from build123d import *

# Parameters (mm, degrees)
F0_R     = 2.75
F1_DEPTH = 7.5
F2_R     = 2


with BuildPart() as f1:
    # F0 (on Top) → F1 (new body)
    with BuildSketch(Plane.XY):
        with BuildLine():
            Line((23.5, 40), (-23.5, 40))
            ThreePointArc((-23.5, 40), (-27.035534, 38.535534), (-28.5, 35))
            Line((-28.5, 35), (-28.5, -35))
            ThreePointArc((-28.5, -35), (-27.035534, -38.535534), (-23.5, -40))
            Line((-23.5, -40), (23.5, -40))
            ThreePointArc((23.5, -40), (27.035534, -38.535534), (28.5, -35))
            Line((28.5, -35), (28.5, 35))
            ThreePointArc((28.5, 35), (27.035534, 38.535534), (23.5, 40))
        make_face()
        with Locations((-23.5, -30)):
            Circle(F0_R, mode=Mode.SUBTRACT)
        with Locations((23.5, -30)):
            Circle(F0_R, mode=Mode.SUBTRACT)
        with Locations((-23.5, 0)):
            Circle(F0_R, mode=Mode.SUBTRACT)
        with Locations((-23.5, 30)):
            Circle(F0_R, mode=Mode.SUBTRACT)
        with BuildLine():
            ThreePointArc((-18.5, 33), (-17.914214, 34.414214), (-16.5, 35))
            Line((-16.5, 35), (16.5, 35))
            ThreePointArc((16.5, 35), (17.914214, 34.414214), (18.5, 33))
            Line((18.5, 33), (18.5, -33))
            ThreePointArc((18.5, -33), (17.914214, -34.414214), (16.5, -35))
            Line((16.5, -35), (-16.5, -35))
            ThreePointArc((-16.5, -35), (-17.914214, -34.414214), (-18.5, -33))
            Line((-18.5, -33), (-18.5, 33))
        make_face(mode=Mode.SUBTRACT)
        with Locations((23.5, 0)):
            Circle(F0_R, mode=Mode.SUBTRACT)
        with Locations((23.5, 30)):
            Circle(F0_R, mode=Mode.SUBTRACT)
    extrude(amount=F1_DEPTH)

    # F2
    f2_edges = [f1.edges().sort_by_distance(p)[0] for p in [
        (-18.5, 0, 7.5),
        (0, -40, 7.5),
    ]]
    fillet(f2_edges, radius=F2_R)


solid = f1.part
Here's how the part is built. I have some questions about the finished solid (model axes, mm). A direction names the side the tool comes from. Round coordinates to 2 decimals unless told otherwise and drop trailing zeros. Write each loop counter-clockwise with the first axis right and the second up, starting at its lowest first coordinate (ties: lowest second). Pieces come first, ordered by that corner, then holes.
1. I need wall thicknesses on L1, parallel to Y at x = -23.5, z = 5.5; L2, parallel to X at y = 22, z = 3; L3, parallel to X at y = 32, z = 4.5. Which ranges of each line are inside material? Lowest first, please.
2. Suppose I cut it at C-C (y = -30). List the corners of the cut face in (x, z) for me, and give its area (3 significant figures).
3. Suppose I cut it at B-B (y = -12). List the corners of the cut face in (x, z) for me, and give its area (3 significant figures).
4. If we mould it in two halves opening along Y, with no side actions, what happens to faces 1 (the cylindrical face through (-0.33, 39.43, 6.9)), 2 (the cylindrical face through (17.93, -34.4, 2.71)), 3 (the cylindrical face through (-26.247, 0.121, 3.698)), 4 (the flat face through (28.5, 0, 3))? For each: released by +Y, released by -Y, zero draft, split by the parting line, or undercut.
5. For faces 5 (the cylindrical face through (17.9, 34.43, 2.71)), 6 (the cylindrical face through (27.07, 38.5, 2.71)), 7 (the cylindrical face through (0.23, 35.57, 6.9)), which set-ups out of +Z, -Z, +X, -X, +Y, -Y let a thin tool reach every point of the face, with its end or its side?
6. Suppose I cut it at D-D (x = 25). State how many separate pieces and enclosed holes the cut face has, and give its area (3 significant figures).
7. Suppose I cut it at A-A (x = 13). List the corners of the cut face in (y, z) for me, and give its area (3 significant figures).
Answer sheet:
1. L1: y = -40 to -32.75, -27.25 to -2.75, 2.75 to 27.25, 32.75 to 40
1. L2: x = -28.5 to -18.5, 18.5 to 28.5
1. L3: x = -28.5 to -25.39, -21.61 to -18.5, 18.5 to 21.61, 25.39 to 28.5
2. outline: (-28.5, 0) - (-26.25, 0) - (-26.25, 7.5) - (-26.5, 7.5) arc R2 ccw to (-28.5, 5.5) - close; (-20.75, 0) - (-18.5, 0) - (-18.5, 5.5) arc R2 ccw to (-20.5, 7.5) - (-20.75, 7.5) - close; (18.5, 0) - (20.75, 0) - (20.75, 7.5) - (20.5, 7.5) arc R2 ccw to (18.5, 5.5) - close; (26.25, 0) - (28.5, 0) - (28.5, 5.5) arc R2 ccw to (26.5, 7.5) - (26.25, 7.5) - close
2. area: 64.1 mm2
3. outline: (-28.5, 0) - (-18.5, 0) - (-18.5, 5.5) arc R2 ccw to (-20.5, 7.5) - (-26.5, 7.5) arc R2 ccw to (-28.5, 5.5) - close; (18.5, 0) - (28.5, 0) - (28.5, 5.5) arc R2 ccw to (26.5, 7.5) - (20.5, 7.5) arc R2 ccw to (18.5, 5.5) - close
3. area: 147 mm2
4. face 1: released by +Y
4. face 2: undercut
4. face 3: undercut
4. face 4: zero draft
5. face 5: +Z, -Z
5. face 6: +Z, -Z, +X, +Y
5. face 7: +Z
6. separate pieces: 4
6. enclosed holes: 0
6. area: 491 mm2
7. outline: (-40, 0) - (-35, 0) - (-35, 5.5) arc R2 ccw to (-37, 7.5) - (-38, 7.5) arc R2 ccw to (-40, 5.5) - close; (35, 0) - (40, 0) - (40, 5.5) arc R2 ccw to (38, 7.5) - (37, 7.5) arc R2 ccw to (35, 5.5) - close
7. area: 71.6 mm2
